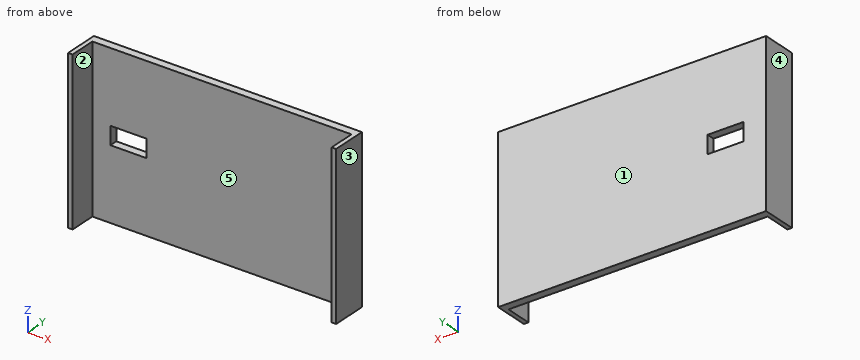
```python
from build123d import *

# Parameters (mm, degrees)
SKETCH1_W           = 300
SKETCH1_H           = 180
BOSS_EXTRUDE1_DEPTH = 9
SKETCH2_W           = 5
SKETCH2_H           = 180
BOSS_EXTRUDE2_DEPTH = 30
SKETCH3_W           = 40.3
SKETCH3_H           = 20
CUT_EXTRUDE1_DEPTH  = 9


with BuildPart() as part:
    # Sketch1 → Boss-Extrude1 (new body)
    with BuildSketch(Plane(origin=(0, 0, 0), x_dir=(1, 0, 0), z_dir=(0, 1, 0))):
        with Locations((150, 90)):
            Rectangle(SKETCH1_W, SKETCH1_H)
    extrude(amount=BOSS_EXTRUDE1_DEPTH)

    # Sketch2 → Boss-Extrude2 (add)
    with BuildSketch(Plane.XZ):
        with Locations((2.5, -90)):
            Rectangle(SKETCH2_W, SKETCH2_H)
        with Locations((297.5, -90)):
            Rectangle(SKETCH2_W, SKETCH2_H)
    extrude(amount=BOSS_EXTRUDE2_DEPTH)

    # Sketch3 → Cut-Extrude1 (cut)
    with BuildSketch(Plane(origin=(0, 9, 0), x_dir=(1, 0, 0), z_dir=(0, 1, 0))):
        with Locations((45.35, 90)):
            Rectangle(SKETCH3_W, SKETCH3_H)
    extrude(amount=-CUT_EXTRUDE1_DEPTH, mode=Mode.SUBTRACT)


solid = part.part
```
Input: part model. Units: mm. Frame: model coordinates. Face numbers are marked on the shaded views. A direction names the side the tool comes from. Coordinates: 2 decimals unless noted, no trailing zeros. Loops run counter-clockwise (first coordinate to the right, second up) from the corner with the lowest first, then second, coordinate; pieces in that order, holes last.
Q1. Mould query, pull axis X, two halves, no side actions, for the marked faces 3, 4 and 5. Classes: +X half, -X half, draft (parallel to the pull), parting line (faces both ways), or undercut.
Results are:
face 3: +X half
face 4: -X half
face 5: undercut
Q2. Contact query for a flat-ended pin moving along its axis: pin 1 (5 mm diameter, centred on x = 154.5, z = -35.5, fed in from -Y). Output: stop coordinate, or through.
Results are:
pin 1: stops at y = 0
Q3. Line query: line 1 along X through (y, z) = (2, -95.5); line 2 along X through (y, z) = (-18, -132.5); line 3 along Y through (x, z) = (94, -118). Output: solid intervals per line, ascending.
Results are:
line 1: x = 0 to 25.2, 65.5 to 300
line 2: x = 0 to 5, 295 to 300
line 3: y = 0 to 9
Q4. Section A-A, the plane y = -16. Return the cut outline in (x, z), and give its area (3 significant figures).
Results are:
outline: (0, -180) - (5, -180) - (5, 0) - (0, 0) - close; (295, -180) - (300, -180) - (300, 0) - (295, 0) - close
area: 1,800 mm2
Q5. Section D-D, the plane x = 124. Return the cut outline in (y, z), and give its area (3 significant figures).
Results are:
outline: (0, -180) - (9, -180) - (9, 0) - (0, 0) - close
area: 1,620 mm2
Q6. Section C-C, the plane z = -144. Return the cut outline in (x, y).
Results are:
outline: (0, -30) - (5, -30) - (5, 0) - (295, 0) - (295, -30) - (300, -30) - (300, 9) - (0, 9) - close
Q7. Set-up query: the marked faces 1 and 2. Return all of +Z, -Z, +X, -X, +Y, -Y with unobstructed straight access to the full face (end or side cutting, diameter ignored); none if empty.
Results are:
face 1: +Z, -Z, +X, -X, +Y
face 2: +Z, -Z, -Y
Q8. Section B-B, the plane z = -92.5. Return the cut outline in (x, y).
Results are:
outline: (0, -30) - (5, -30) - (5, 0) - (25.2, 0) - (25.2, 9) - (0, 9) - close; (65.5, 0) - (295, 0) - (295, -30) - (300, -30) - (300, 9) - (65.5, 9) - close
